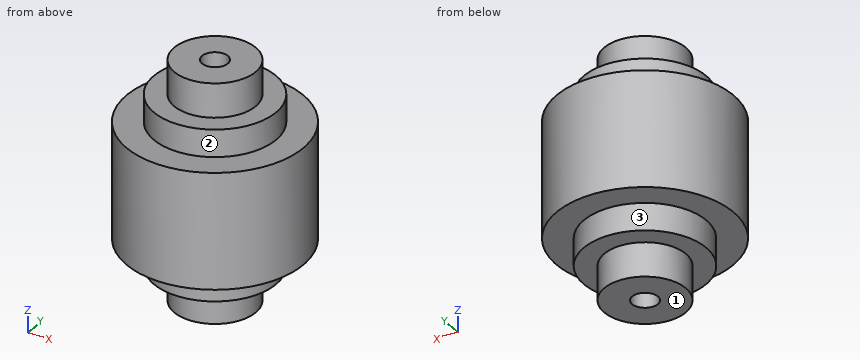
from build123d import *

# Parameters (mm, degrees)
SKETCH_2_R           = 1.9
CUT_EXTRUDE_1_DEPTH  = 36
EXTRUDE_1_DEPTH      = 4
EXTRUDE_1_DEPTH_BACK = 21
SKETCH_4_R           = 9


with BuildPart() as part:
    # 草图1 → 旋转1 (revolve)
    with BuildSketch(Plane(origin=(0, 0, 0), x_dir=(1, 0, 0), z_dir=(0, 1, 0)), mode=Mode.PRIVATE) as revolve_1_sk:
        Polygon((0, -1e-09), (0, -35), (6, -35), (6, -30), (7.5, -30), (7.5, -26), (9, -26), (13, -26), (13, -9), (9, -9), (7.5, -9), (7.5, -5), (6, -5), (6, -1e-09), align=None)
    revolve(revolve_1_sk.sketch.rotate(Axis((0, 0, 1e-09), (0, 0, 1)), 180), axis=Axis((0, 0, 1e-09), (0, 0, 1)))

    # 草图2 → 切除-拉伸1 (cut)
    with BuildSketch(Plane.XY.offset(35)):
        Circle(SKETCH_2_R)
    extrude(amount=-CUT_EXTRUDE_1_DEPTH, mode=Mode.SUBTRACT)

    # 草图4 → 凸台-拉伸1 (add, two sides: drawn at the far end of the back side and taken through both)
    with BuildSketch(Plane.XY.offset(26).offset(-EXTRUDE_1_DEPTH_BACK)):
        Circle(SKETCH_4_R)
    extrude(amount=EXTRUDE_1_DEPTH + EXTRUDE_1_DEPTH_BACK)


solid = part.part
Source: CAD feature listing. Evaluate the final solid. Frame: model axes, mm. Face numbers are marked on the shaded views. A direction names the side the tool comes from. Round coordinates to 2 decimals unless told otherwise and drop trailing zeros. Loops run counter-clockwise (first coordinate to the right, second up) from the corner with the lowest first, then second, coordinate; pieces in that order, holes last. Notation, with made-up numbers: M -31,8 L -7,8 A19 ccw -7,23 Z; hole C 9.25,66 d3. An arc over 180 degrees is marked long. Return JSON: item names as keys, results as strings. Group by question number.
1. Section query D-D on y = -4.25. Output: boundary loops of the cut face in (x, z).
2. Section query A-A on y = 0. Output: boundary loops of the cut face in (x, z).
3. Section query C-C on z = 24. Output: boundary loops of the cut face in (x, y), and give its area (3 significant figures).
4. Reachability of the marked faces 1, 2 and 3 from +Z, -Z, +X, -X, +Y, -Y: full face, straight path, thin tool, end or side. Return the list, or none.
5. Material intervals for line 1 along Y through (x, z) = (0, 2.8); line 2 along Z through (x, y) = (7.5, 10.5); line 3 along Z through (x, y) = (-0.5, 6.25), sorted ascending. Write a range as from..to.
6. Pin query (flat end, axial travel): pin 1 (3 mm diameter, centred on x = 0, y = 0, fed in from +Z); pin 2 (1.9 mm diameter, centred on x = 0, y = 0.5, fed in from -Z); pin 3 (1 mm diameter, centred on x = 6.5, y = -10, fed in from +Z). Return the tip coordinate at first contact, or that it passes through.
Checks:
{
 "1": {"outline": "M -12.29,9 L -7.93,9 L -7.93,5 L -4.24,5 L -4.24,0 L 4.24,0 L 4.24,5 L 7.93,5 L 7.93,9 L 12.29,9 L 12.29,26 L 7.93,26 L 7.93,30 L 4.24,30 L 4.24,35 L -4.24,35 L -4.24,30 L -7.93,30 L -7.93,26 L -12.29,26 Z"},
 "2": {"outline": "M -13,9 L -9,9 L -9,5 L -6,5 L -6,0 L -1.9,0 L -1.9,5 L 1.9,5 L 1.9,0 L 6,0 L 6,5 L 9,5 L 9,9 L 13,9 L 13,26 L 9,26 L 9,30 L 6,30 L 6,35 L 1.9,35 L 1.9,30 L -1.9,30 L -1.9,35 L -6,35 L -6,30 L -9,30 L -9,26 L -13,26 Z"},
 "3": {"outline": "C 0,0 d26", "area": "531 mm²"},
 "4": {"face 1": "-Z, +X, -X, +Y, -Y", "face 2": "+Z", "face 3": "-Z"},
 "5": {"line 1": "y = -6..-1.9, 1.9..6", "line 2": "z = 9..26", "line 3": "z = 5..30"},
 "6": {"pin 1": "stops at z = 30", "pin 2": "stops at z = 5", "pin 3": "stops at z = 26"}
}
